Verification items for this drawing (mm, ordinates from the low corner). Round coordinates to 2 decimals unless told otherwise and drop trailing zeros. Order: outer loops, then holes, each group sorted by start corner. A loop starts at its lowest first (then second) coordinate and runs counter-clockwise, first axis right, second up. Notation, with made-up numbers: (30, -30.75) -> (38, -30.75) arc R21 cw to (38, -15.75) -> close; hole circle Ø5 at (80, 58). An arc over 180 degrees is marked (long way). Put each result on its own line as item: value.
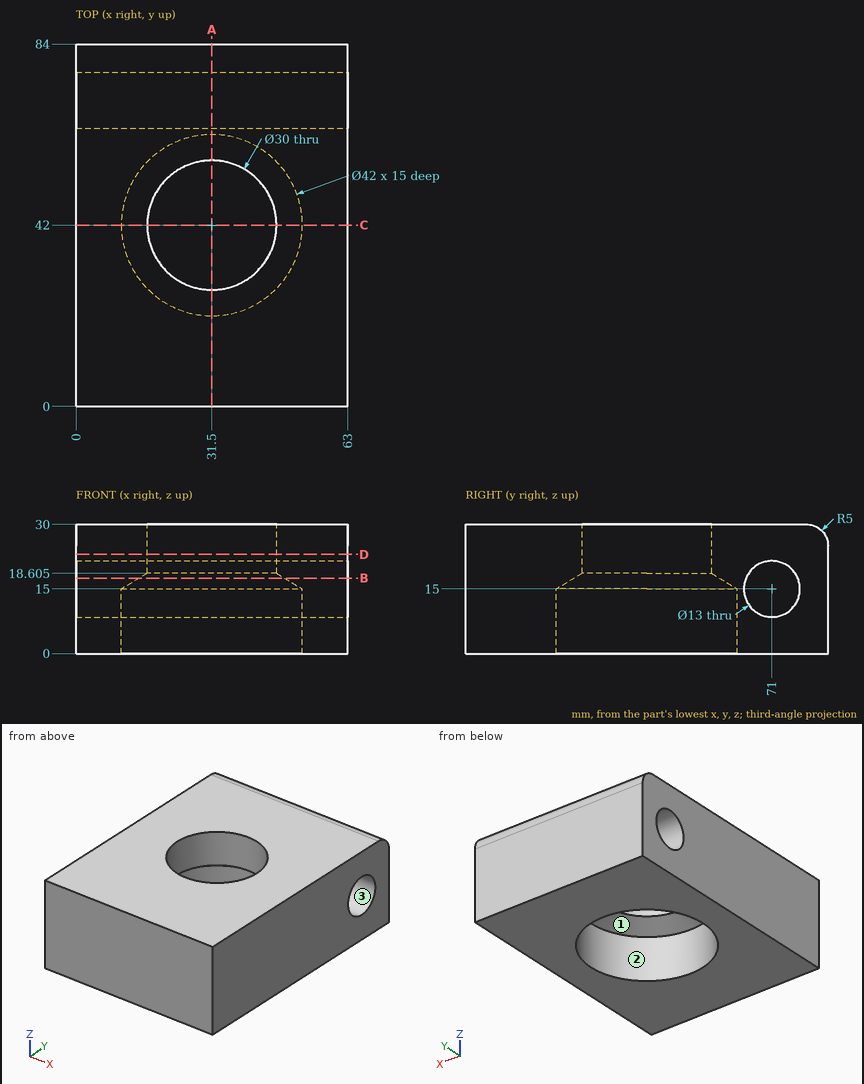
Item 1: Release check for a two-part mould opening along Z. For the marked faces 1, 2 and 3 record: +Z half, -Z half, draft (parallel to the pull), parting line (faces both ways), or undercut.
Check sheet entries:
face 1: -Z half
face 2: draft
face 3: undercut
Item 2: Section check A-A on x = 31.5. Record the boundary of the cut face in (y, z) (1 decimal).
Check sheet entries:
outline: (0, 0) -> (21, 0) -> (21, 15) -> (27, 18.6) -> (27, 30) -> (0, 30) -> close; (57, 18.6) -> (63, 15) -> (63, 0) -> (84, 0) -> (84, 25) arc R5 ccw to (79, 30) -> (57, 30) -> close; hole circle Ø13 at (71, 15)
Item 3: Section check D-D on z = 23. Record the boundary of the cut face in (x, y), then the cut area to 3 significant figures.
Check sheet entries:
outline: (0, 0) -> (63, 0) -> (63, 84) -> (0, 84) -> close; hole circle Ø30 at (31.5, 42)
area: 4,590 mm^2
Item 4: Section check B-B on z = 17.5. Record the boundary of the cut face in (x, y).
Check sheet entries:
outline: (0, 0) -> (63, 0) -> (63, 65) -> (0, 65) -> close; (0, 77) -> (63, 77) -> (63, 84) -> (0, 84) -> close; hole circle Ø33.68 at (31.5, 42)
Item 5: Section check C-C on y = 42. Record the boundary of the cut face in (x, z) (1 decimal), then the cut area to 3 significant figures.
Check sheet entries:
outline: (0, 0) -> (10.5, 0) -> (10.5, 15) -> (16.5, 18.6) -> (16.5, 30) -> (0, 30) -> close; (46.5, 18.6) -> (52.5, 15) -> (52.5, 0) -> (63, 0) -> (63, 30) -> (46.5, 30) -> close
area: 788 mm^2
Item 6: Material ranges on L1, parallel to Y at x = 31.5, z = 8.25; L2, parallel to Y at x = 31.5, z = 24; L3, parallel to X at y = 53, z = 22, recorded low to high. Write a range as [from, to].
Check sheet entries:
L1: y = [0, 21], [63, 84]
L2: y = [0, 27], [57, 84]
L3: x = [0, 21.3], [41.7, 63]
Item 7: Gauge pin test, flat end, axial feed: pin 1 Ø12 at (x, y) = (48.5, 28) entering from -Z. Record the tip position at first contact, or that the pin passes through.
Check sheet entries:
pin 1: stops at z = 0
